Design review of the part built by this model. Coordinates are the model's own, in mm. Face numbers are marked on the shaded views. A direction names the side the tool comes from. Coordinates: 2 decimals unless noted, no trailing zeros. Order: outer loops, then holes, each group sorted by start corner. A loop starts at its lowest first (then second) coordinate and runs counter-clockwise, first axis right, second up. Notation, with made-up numbers: (64, -16) -> (104, -16) arc R14 ccw to (104, 5) -> close; hole circle Ø3 at (38.25, 75.5). An arc over 180 degrees is marked (long way). Use a Markdown table: item, result. Add a question column.
Q1. Wall thickness on probe 1 along Y at (x, z) = (8.45, 0); probe 2 along Y at (x, z) = (9.5, -7.5): over which ranges is each line inside the solid? List them lowest first.
Q2. Insertion check: pin 1 (0.9 mm diameter, centred on x = -11.5, y = 1, fed in from +Z); pin 2 (2.5 mm diameter, centred on y = 0, z = 0, fed in from -X); pin 3 (2 mm diameter, centred on x = 6, y = -0.5, fed in from -Z); pin 4 (1.2 mm diameter, centred on x = -11, z = -1, fed in from -Y). Each pin has a flat end and moves straight along its axis. Give the tip position at first contact, or say it passes through.
Q3. Add section B-B (y = 0). Count the separate pieces of the cut face and the enclosed holes in it, then the cut area to 3 significant figures.
Q4. The part is to be moulded in two halves that separate along Y. For the marked faces 1, 2 and 3, say which applies: pulls with the +Y half, pulls with the -Y half, needs draft (parallel to the pull), parting line crosses it, or undercut.
Q5. Add section C-C (y = 8). State the section outline as (x, z) points, then the cut area to 3 significant figures.
Q6. Add section D-D (x = -2.5). State the section outline as (y, z) points.
Q7. Machinability: for the marked faces 4, 5, 6 and 7, which of the approach directions +Z, -Z, +X, -X, +Y, -Y give a long, thin tool a straight path to every point of the face, cutting with its end or side? Answer none if there is none.
Q8. Add section A-A (x = 6.5). State the section outline as (y, z) points.
from build123d import *

# Parameters (mm, degrees)
SWEEP_1_PROFILE_R        = 1.5
EXTRUDE_1_DEPTH          = 3.44
EXTRUDE_1_DEPTH_BACK     = 4.5
EXTRUDE_1_START          = 9.5
SKETCH_8_R               = 2.5
EXTRUDE_2_DEPTH          = 4.5
EXTRUDE_2_DEPTH_BACK     = 3.44
EXTRUDE_2_START          = -9.5
SKETCH_9_R               = 2.5
EXTRUDE_START            = 9.94
SKETCH_14_R              = 1
EXTRUDE_3_DEPTH          = 2
CUT_EXTRUDE_START        = 12.94
CUT_EXTRUDE_1_DEPTH      = 4
CUT_EXTRUDE_START_2      = -8.94
CUT_EXTRUDE_2_DEPTH      = 4
SKETCH_16_R              = 0.25
CUT_EXTRUDE_3_DEPTH      = 0.25
CUT_EXTRUDE_START_3      = 8.69
SKETCH_17_R              = 0.25
CUT_EXTRUDE_4_DEPTH      = 0.25
EXTRUDE_START_2          = 5
SKETCH_18_R              = 3.5
EXTRUDE_4_DEPTH          = 3.94
EXTRUDE_START_3          = -8.94
SKETCH_20_R              = 3.5
EXTRUDE_5_DEPTH          = 3.94
CUT_EXTRUDE_6_DEPTH      = 19.653246417
CUT_EXTRUDE_6_DEPTH_BACK = 19.653246417
SKETCH_25_R              = 1
FILLET_1_R               = 1
CUT_EXTRUDE_START_4      = -5
CUT_EXTRUDE_7_DEPTH      = 2
CUT_EXTRUDE_START_5      = 5
CUT_EXTRUDE_8_DEPTH      = 2


with BuildPart() as part:
    # 扫描1: sweep along a path in 草图1
    with BuildLine(Plane.XY) as sweep_1_path:
        Line((9.5, 0), (6.5, 0))
        Line((6.5, 0), (6.5, 8))
        Line((6.5, 8), (-6.5, 8))
        Line((-6.5, 8), (-6.5, 0))
        Line((-6.5, 0), (-9.5, 0))
    # 扫描1 profile (on start of the path) → 扫描1 (sweep)
    with BuildSketch(Plane(origin=(9.5, 0, 0), x_dir=(0, -1, 0), z_dir=(-1, 0, 0))):
        Circle(SWEEP_1_PROFILE_R)
    sweep(path=sweep_1_path.line, transition=Transition.RIGHT)

    # 草图8 → 凸台-拉伸1 (add, two sides: drawn at the far end of the back side and taken through both)
    with BuildSketch(Plane(origin=(0, 0, 0), x_dir=(0, 0, -1), z_dir=(1, 0, 0)).offset(EXTRUDE_1_START - EXTRUDE_1_DEPTH_BACK)):
        with Locations(Location((0, 0, 0), (0, 0, 90))):
            Circle(SKETCH_8_R)
    extrude(amount=EXTRUDE_1_DEPTH + EXTRUDE_1_DEPTH_BACK)

    # 草图9 → 凸台-拉伸2 (add, two sides: drawn at the far end of the back side and taken through both)
    with BuildSketch(Plane(origin=(0, 0, 0), x_dir=(0, 0, -1), z_dir=(1, 0, 0)).offset(EXTRUDE_2_START - EXTRUDE_2_DEPTH_BACK)):
        with Locations(Location((0, 0, 0), (0, 0, 90))):
            Circle(SKETCH_9_R)
    extrude(amount=EXTRUDE_2_DEPTH + EXTRUDE_2_DEPTH_BACK)

    # 草图14 → 凸台-拉伸3 (add)
    with BuildSketch(Plane(origin=(0, 0, 0), x_dir=(0, 0, -1), z_dir=(1, 0, 0)).offset(EXTRUDE_START)):
        with BuildLine():
            Line((0.166666667, 2.494438258), (7.633333333, 1.995550606))
            ThreePointArc((7.633333333, 1.995550606), (9.5, 0), (7.633333333, -1.995550606))
            Line((7.633333333, -1.995550606), (0.166666667, -2.494438258))
            ThreePointArc((0.166666667, -2.494438258), (-2.5, 0), (0.166666667, 2.494438258))
        make_face()
        with Locations((7.5, 0)):
            Circle(SKETCH_14_R, mode=Mode.SUBTRACT)
    extrude(amount=-EXTRUDE_3_DEPTH)

    # 草图10 → 切除-拉伸1 (cut)
    with BuildSketch(Plane(origin=(0, 0, 0), x_dir=(0, 0, -1), z_dir=(1, 0, 0)).offset(CUT_EXTRUDE_START)):
        with BuildLine():
            Line((0.75, 0.75), (1.854049622, 0.75))
            ThreePointArc((1.854049622, 0.75), (2, 0), (1.854049622, -0.75))
            Line((1.854049622, -0.75), (0.75, -0.75))
            Line((0.75, -0.75), (0.75, -1.854049622))
            ThreePointArc((0.75, -1.854049622), (0, -2), (-0.75, -1.854049622))
            Line((-0.75, -1.854049622), (-0.75, -0.75))
            Line((-0.75, -0.75), (-1.854049622, -0.75))
            ThreePointArc((-1.854049622, -0.75), (-2, 0), (-1.854049622, 0.75))
            Line((-1.854049622, 0.75), (-0.75, 0.75))
            Line((-0.75, 0.75), (-0.75, 1.854049622))
            ThreePointArc((-0.75, 1.854049622), (0, 2), (0.75, 1.854049622))
            Line((0.75, 1.854049622), (0.75, 0.75))
        make_face()
    extrude(amount=-CUT_EXTRUDE_1_DEPTH, mode=Mode.SUBTRACT)

    # 草图11 → 切除-拉伸2 (cut)
    with BuildSketch(Plane(origin=(0, 0, 0), x_dir=(0, 0, -1), z_dir=(1, 0, 0)).offset(CUT_EXTRUDE_START_2)):
        with BuildLine():
            Line((0.75, 0.75), (0.75, 1.854049622))
            ThreePointArc((0.75, 1.854049622), (0, 2), (-0.75, 1.854049622))
            Line((-0.75, 1.854049622), (-0.75, 0.75))
            Line((-0.75, 0.75), (-1.854049622, 0.75))
            ThreePointArc((-1.854049622, 0.75), (-2, 0), (-1.854049622, -0.75))
            Line((-1.854049622, -0.75), (-0.75, -0.75))
            Line((-0.75, -0.75), (-0.75, -1.854049622))
            ThreePointArc((-0.75, -1.854049622), (0, -2), (0.75, -1.854049622))
            Line((0.75, -1.854049622), (0.75, -0.75))
            Line((0.75, -0.75), (1.854049622, -0.75))
            ThreePointArc((1.854049622, -0.75), (2, 0), (1.854049622, 0.75))
            Line((1.854049622, 0.75), (0.75, 0.75))
        make_face()
    extrude(amount=-CUT_EXTRUDE_2_DEPTH, mode=Mode.SUBTRACT)

    # 草图16 → 切除-拉伸3 (cut)
    with BuildSketch(Plane(origin=(0, 0, 0), x_dir=(0, 0, -1), z_dir=(1, 0, 0)).offset(CUT_EXTRUDE_START_2)):
        with Locations(Location((0.75, 0, 0), (0, 0, 90))):
            Circle(SKETCH_16_R)
    extrude(amount=CUT_EXTRUDE_3_DEPTH, mode=Mode.SUBTRACT)

    # 草图17 → 切除-拉伸4 (cut)
    with BuildSketch(Plane(origin=(0, 0, 0), x_dir=(0, 0, -1), z_dir=(1, 0, 0)).offset(CUT_EXTRUDE_START_3)):
        with Locations(Location((0.75, 0, 0), (0, 0, 90))):
            Circle(SKETCH_17_R)
    extrude(amount=CUT_EXTRUDE_4_DEPTH, mode=Mode.SUBTRACT)

    # 草图18 → 凸台-拉伸4 (add)
    with BuildSketch(Plane(origin=(0, 0, 0), x_dir=(0, 0, -1), z_dir=(1, 0, 0)).offset(EXTRUDE_START_2)):
        with Locations(Location((0, 0, 0), (0, 0, 90))):
            Circle(SKETCH_18_R)
    extrude(amount=EXTRUDE_4_DEPTH)

    # 草图20 → 凸台-拉伸5 (add)
    with BuildSketch(Plane(origin=(0, 0, 0), x_dir=(0, 0, -1), z_dir=(1, 0, 0)).offset(EXTRUDE_START_3)):
        with Locations(Location((0, 0, 0), (0, 0, 90))):
            Circle(SKETCH_20_R)
    extrude(amount=EXTRUDE_5_DEPTH)

    # 草图25 → 切除-拉伸6 (cut, two sides: drawn at the far end of the back side and taken through both)
    with BuildSketch(Plane(origin=(0, 0, 0), x_dir=(0, 0, -1), z_dir=(1, 0, 0)).offset(-CUT_EXTRUDE_6_DEPTH_BACK)):
        Circle(SKETCH_25_R)
    extrude(amount=CUT_EXTRUDE_6_DEPTH + CUT_EXTRUDE_6_DEPTH_BACK, mode=Mode.SUBTRACT)

    # 圆角1
    # the kernel refuses this fillet: 1 mm, written as the material it adds along each edge
    with BuildSketch(Plane(origin=(-8.94, 0, 0), x_dir=(0, 1, 0), z_dir=(0, 0, 1))) as fillet_1_piece_1:
        with BuildLine():
            CenterArc((2.5 + FILLET_1_R, FILLET_1_R), FILLET_1_R, 180, 90)
            Line((2.5, FILLET_1_R), (2.5, 0))
            Line((2.5, 0), (2.5 + FILLET_1_R, 0))
        make_face()
    revolve(axis=Axis((-8.94, 0, 0), (-1, 0, 0)))
    with BuildSketch(Plane(origin=(8.94, 0, 0), x_dir=(0, 1, 0), z_dir=(0, 0, -1))) as fillet_1_piece_2:
        with BuildLine():
            CenterArc((2.5 + FILLET_1_R, FILLET_1_R), FILLET_1_R, 180, 90)
            Line((2.5 + FILLET_1_R, 0), (2.5, 0))
            Line((2.5, 0), (2.5, FILLET_1_R))
        make_face()
    revolve(axis=Axis((8.94, 0, 0), (1, 0, 0)), revolution_arc=183.822553729)
    with BuildSketch(Plane(origin=(8.94, -2.494438258, -0.166666667), x_dir=(1, 0, 0), z_dir=(0, 0.06666666666666658, -0.9977753031397177))) as fillet_1_piece_3_section:
        with BuildLine():
            CenterArc((FILLET_1_R, FILLET_1_R), FILLET_1_R, 180, 90)
            Line((0, FILLET_1_R), (0, 0))
            Line((0, 0), (FILLET_1_R, 0))
        make_face()
    fillet_1_piece_3 = extrude(amount=4.949489743, mode=Mode.PRIVATE)
    fillet_1_piece_3 = fillet_1_piece_3 & Plane(origin=(9.184299624, 0, 0), x_dir=(0, 1, 0), z_dir=(-1, 0, 0)) * Cylinder(3.5, 14, mode=Mode.PRIVATE)
    add(fillet_1_piece_3)
    with BuildSketch(Plane(origin=(8.94, 2.164472275, -5.105145295), x_dir=(0, 0.9977753031397177, -0.0666666666666666), z_dir=(0, 0.06666666666666658, 0.9977753031397177))) as fillet_1_piece_4_section:
        with BuildLine():
            CenterArc((FILLET_1_R, -FILLET_1_R), FILLET_1_R, 90, 90)
            Line((0, -FILLET_1_R), (0, 0))
            Line((0, 0), (FILLET_1_R, 0))
        make_face()
    fillet_1_piece_4 = extrude(amount=4.949489743, mode=Mode.PRIVATE)
    fillet_1_piece_4 = fillet_1_piece_4 & Plane(origin=(9.184299625, 0, 0), x_dir=(0, 1, 0), z_dir=(-1, 0, 0)) * Cylinder(3.5, 14, mode=Mode.PRIVATE)
    add(fillet_1_piece_4)
    with BuildSketch(Plane(origin=(8.94, 0, 0), x_dir=(0, 0.9977753030864385, -0.06666666746407793), z_dir=(0, -0.06666666746407793, -0.9977753030864385))) as fillet_1_piece_5:
        with BuildLine():
            CenterArc((2.5 + FILLET_1_R, FILLET_1_R), FILLET_1_R, 180, 90)
            Line((2.5, FILLET_1_R), (2.5, 0))
            Line((2.5, 0), (2.5 + FILLET_1_R, 0))
        make_face()
    revolve(axis=Axis((8.94, 0, 0), (1, 0, 0)), revolution_arc=3.822553775)

    # 草图26 → 切除-拉伸7 (cut)
    with BuildSketch(Plane(origin=(0, 0, 0), x_dir=(0, 0, -1), z_dir=(1, 0, 0)).offset(CUT_EXTRUDE_START_4)):
        Polygon((0, -2.309401077), (2, -1.154700538), (2, 1.154700538), (0, 2.309401077), (-2, 1.154700538), (-2, -1.154700538), align=None)
    extrude(amount=-CUT_EXTRUDE_7_DEPTH, mode=Mode.SUBTRACT)

    # 草图27 → 切除-拉伸8 (cut)
    with BuildSketch(Plane(origin=(0, 0, 0), x_dir=(0, 0, -1), z_dir=(1, 0, 0)).offset(CUT_EXTRUDE_START_5)):
        Polygon((0, -2.309401077), (2, -1.154700538), (2, 1.154700538), (0, 2.309401077), (-2, 1.154700538), (-2, -1.154700538), align=None)
    extrude(amount=CUT_EXTRUDE_8_DEPTH, mode=Mode.SUBTRACT)


solid = part.part
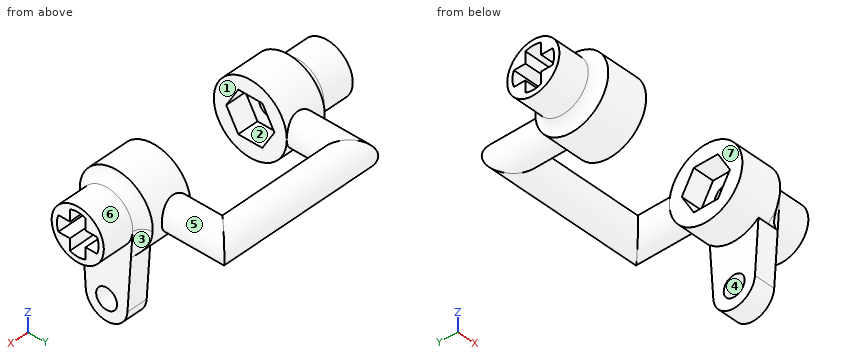
Established:
| question | item | result |
|---|---|---|
| 1 | probe 1 | -3.5 to -1, 1 to 3.5 |
| 1 | probe 2 | -2 to -1, 1 to 2 |
| 2 | pin 1 | z = 2.44 |
| 2 | pin 2 | x = -12.94 |
| 2 | pin 3 | z = -3.5 |
| 2 | pin 4 | y = -2.47 |
| 3 | separate pieces | 5 |
| 3 | enclosed holes | 0 |
| 3 | area | 49.0 mm^2 |
| 4 | face 1 | needs draft |
| 4 | face 2 | undercut |
| 4 | face 3 | pulls with the +Y half |
| 5 | outline | (-6.5, -1.5) -> (6.5, -1.5) arc R1.5 ccw to (6.5, 1.5) -> (-6.5, 1.5) arc R1.5 ccw to start |
| 5 | area | 46.1 mm^2 |
| 6 | outline | circle Ø3 at (8, 0) |
| 7 | face 4 | +X, -X |
| 7 | face 5 | none |
| 7 | face 6 | +X |
| 7 | face 7 | +Z, -Z, -Y |
| 8 | outline | (3.16, -1.5) -> (8, -1.5) arc R1.5 ccw to (8, 1.5) -> (3.16, 1.5) arc R3.5 ccw (long way) to start; hole (-2.31, 0) -> (-1.15, -2) -> (1.15, -2) -> (2.31, 0) -> (1.15, 2) -> (-1.15, 2) -> close |
